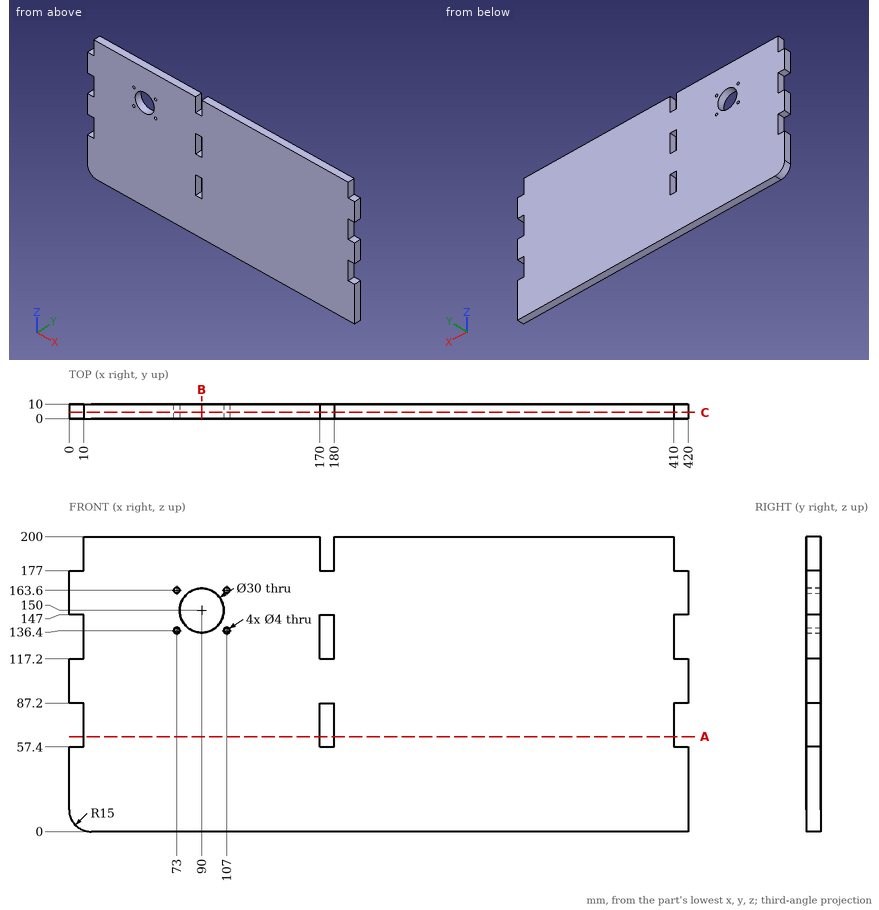
Geometry check sheet. Reference: drawing and pictorial views, mm from the part's lowest x, y, z. Give positions to 0.01 mm unless a question says otherwise; leave off trailing zeros. Write each loop counter-clockwise with the first axis right and the second up, starting at its lowest first coordinate (ties: lowest second). Pieces come first, ordered by that corner, then holes. Notation, with made-up numbers: (-22.5, -39) - (2.5, -39) arc R20 cw to (2.5, -11) - close; hole circle Ø10 at (10.25, 78.25). An arc over 180 degrees is marked (long way). Use a Markdown table: item, result.
Q1. Go/stop test with flat-tipped pins: P1, Ø5, axis at x = 4, y = 5.5, coming from the +Z side; P2, Ø6, axis at x = 178.5, y = 7, coming from the +Z side; P3, Ø5, axis at y = 5.5, z = 135, coming from the -X side; P4, Ø1, axis at y = 4, z = 143, coming from the +X side. Record where each tip stops, or that it passes through.
Computed:
| item | result |
|---|---|
| P1 | stops at z = 177 |
| P2 | stops at z = 200 |
| P3 | stops at x = 10 |
| P4 | stops at x = 410 |
Q2. Thickness scan on L1, parallel to X at y = 8.5, z = 191.5; L2, parallel to Z at x = 90, y = 6.5; L3, parallel to Z at x = 107, y = 5.25. Record the ranges inside material, lowest first. Write a range as [from, to].
Computed:
| item | result |
|---|---|
| L1 | x = [10, 170], [180, 410] |
| L2 | z = [0, 135], [165, 200] |
| L3 | z = [0, 134.4], [138.4, 161.6], [165.6, 200] |
Q3. Section check B-B, the plane x = 90. Enter the section's corners in (y, z).
Computed:
| item | result |
|---|---|
| outline | (0, 0) - (10, 0) - (10, 135) - (0, 135) - close; (0, 165) - (10, 165) - (10, 200) - (0, 200) - close |
Q4. Section check C-C, the plane y = 4.25. Give the number of separate pieces and of enclosed holes in the cut face, then the cut area to 3 significant figures.
Computed:
| item | result |
|---|---|
| separate pieces | 1 |
| enclosed holes | 7 |
| area | 80,700 mm² |
Q5. Section check A-A, the plane z = 64.5. Enter the section's corners in (x, y), then the cut area to 3 significant figures.
Computed:
| item | result |
|---|---|
| outline | (10, 0) - (170, 0) - (170, 10) - (10, 10) - close; (180, 0) - (410, 0) - (410, 10) - (180, 10) - close |
| area | 3,900 mm² |
